Verification items for the finished model (mm, model axes). Face numbers are marked on the shaded views. A direction names the side the tool comes from. Round coordinates to 2 decimals unless told otherwise and drop trailing zeros. Write each loop counter-clockwise with the first axis right and the second up, starting at its lowest first coordinate (ties: lowest second). Pieces come first, ordered by that corner, then holes. Notation, with made-up numbers: (40.5, 44.25) - (60.5, 44.25) arc R22 cw to (60.5, 73.25) - close; hole circle Ø8 at (63.25, -37). An arc over 180 degrees is marked (long way). Answer as a JSON object with one key per item and string values. Group by question number.
1) Section check A-A (y = 4). Enter the section's corners in (x, z) (3 decimals).
2) Section check C-C (y = -8.5). Enter the section's corners in (x, z) (3 decimals), then the cut area to 4 significant figures.
3) Section check D-D (z = -8.5). Enter the section's corners in (x, y), then the cut area to 3 significant figures.
4) Go/stop test with flat-tipped pins: pin 1 Ø4 at (x, z) = (3.5, 12) entering from -Y; pin 2 Ø10 at (x, z) = (8, 4.5) entering from +Y; pin 3 Ø3 at (x, y) = (-26, 3.5) entering from -Z. Record where each tip stops, or that it passes through.
5) Thickness scan on line 1 (X direction, y = 0, z = 21) (3 decimals); line 2 (X direction, y = 5, z = 0) (3 decimals). Record the ranges inside material, lowest first.
6) Mould release check, pull along Z, two halves, no side actions. Record for the marked faces 6, 7 and 8: +Z half, -Z half, draft (parallel to the pull), parting line (faces both ways), or undercut.
7) Section check B-B (z = 10). Enter the section's corners in (x, y).
8) Set-up check for the marked faces 1, 2, 3, 4 and 5: record each of +Z, -Z, +X, -X, +Y, -Y from which the full face is reachable in a straight line by a thin tool's end or side.
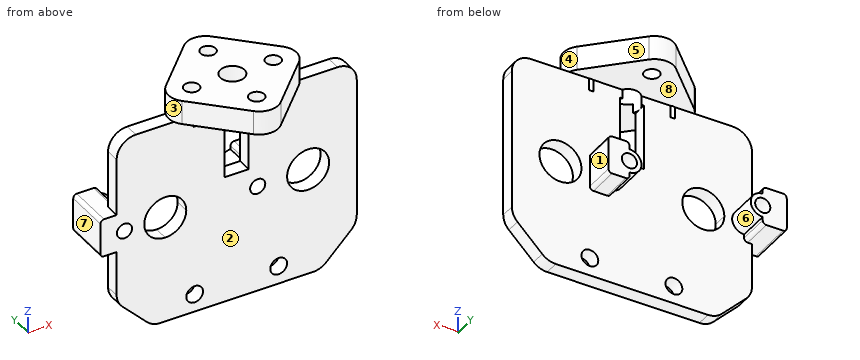
```python
from build123d import *

# Parameters (mm, degrees)
BOSS_EXTRUDE1_DEPTH      = 1.5
BOSS_EXTRUDE1_DEPTH_BACK = 1.5
SKETCH1_W                = 5
SKETCH1_H                = 13.727853371
SKETCH1_R                = 4.375
SKETCH1_R_2              = 1.75
BOSS_EXTRUDE2_DEPTH      = 15
BOSS_EXTRUDE2_DEPTH_BACK = 15
SKETCH2_R                = 1.575
SKETCH2_R_2              = 2.5
CUT_EXTRUDE1_DEPTH       = 7.5
CUT_EXTRUDE2_DEPTH       = 5
BOSS_EXTRUDE3_DEPTH      = 8
BOSS_EXTRUDE3_DEPTH_BACK = 1.5
SKETCH1_4_R              = 1.575
FILLET1_R                = 4
FILLET2_R                = 0.75


with BuildPart() as part:
    # Sketch1 → Boss-Extrude1 (new, two sides: drawn at the far end of the back side and taken through both)
    with BuildSketch(Plane(origin=(0, 0, 0), x_dir=(1, 0, 0), z_dir=(0, 1, 0)).offset(-BOSS_EXTRUDE1_DEPTH_BACK)):
        with BuildLine():
            ThreePointArc((-23.375, 2.5), (-21.607233047, 1.767766953), (-20.875, 0))
            ThreePointArc((-20.875, 0), (-21.607233047, -1.767766953), (-23.375, -2.5))
            Line((-23.375, -2.5), (-23.375, -4))
            Line((-23.375, -4), (-25, -4))
            Line((-25, -4), (-25, -20))
            Line((-25, -20), (25, -20))
            Line((25, -20), (25, 15))
            Line((25, 15), (17.5, 22.5))
            Line((17.5, 22.5), (-17.5, 22.5))
            Line((-17.5, 22.5), (-25, 15))
            Line((-25, 15), (-25, 4))
            Line((-25, 4), (-23.375, 4))
            Line((-23.375, 4), (-23.375, 2.5))
        make_face()
        with Locations((0, -11.238926686)):
            Rectangle(SKETCH1_W, SKETCH1_H, mode=Mode.SUBTRACT)
        with BuildLine():
            ThreePointArc((-10.5, 0), (-14.875, -4.375), (-19.25, 0))
            ThreePointArc((-19.25, 0), (-17.968592168, 3.093592168), (-14.875, 4.375))
            ThreePointArc((-14.875, 4.375), (-11.781407832, 3.093592168), (-10.5, 0))
        make_face(mode=Mode.SUBTRACT)
        with BuildLine():
            ThreePointArc((4.375, -2.5), (2.607233047, -1.767766953), (1.875, 0))
            ThreePointArc((1.875, 0), (2.607233047, 1.767766953), (4.375, 2.5))
            Line((4.375, 2.5), (4.375, 4))
            Line((4.375, 4), (8.75, 4))
            Line((8.75, 4), (8.75, 0))
            Line((8.75, 0), (8.75, -4))
            Line((8.75, -4), (4.375, -4))
            Line((4.375, -4), (4.375, -2.5))
        make_face(mode=Mode.SUBTRACT)
        with Locations(Location((14.875, 0, 0), (0, 0, 270))):
            Circle(SKETCH1_R, mode=Mode.SUBTRACT)
        with Locations(Location((-8.75, 18.75, 0), (0, 0, 270))):
            Circle(SKETCH1_R_2, mode=Mode.SUBTRACT)
        with Locations(Location((8.75, 18.75, 0), (0, 0, 270))):
            Circle(SKETCH1_R_2, mode=Mode.SUBTRACT)
    extrude(amount=BOSS_EXTRUDE1_DEPTH + BOSS_EXTRUDE1_DEPTH_BACK)

    # Sketch1<3> → Boss-Extrude2 (add, two sides: drawn at the far end of the back side and taken through both)
    with BuildSketch(Plane(origin=(0, 0, 0), x_dir=(1, 0, 0), z_dir=(0, 1, 0)).offset(-BOSS_EXTRUDE2_DEPTH_BACK)):
        Polygon((0, -20), (-25, -20), (-25, -25), (25, -25), (25, -20), align=None)
    extrude(amount=BOSS_EXTRUDE2_DEPTH + BOSS_EXTRUDE2_DEPTH_BACK)

    # Sketch2 → Cut-Extrude1 (cut)
    with BuildSketch(Plane.XY.offset(25)):
        with Locations((-8.5, 0)):
            Circle(SKETCH2_R)
        Circle(SKETCH2_R_2)
        with Locations((0, 8.5)):
            Circle(SKETCH2_R)
        with Locations((8.5, 0)):
            Circle(SKETCH2_R)
        with Locations((0, -8.5)):
            Circle(SKETCH2_R)
    extrude(amount=-CUT_EXTRUDE1_DEPTH, mode=Mode.SUBTRACT)

    # Sketch2<3> → Cut-Extrude2 (cut)
    with BuildSketch(Plane.XY.offset(25)):
        Polygon((-25, 0), (-15, 0), (0, 15), (-25, 15), align=None)
        Polygon((25, 15), (0, 15), (15, 0), (0, -15), (25, -15), align=None)
        Polygon((0, -15), (-15, 0), (-25, 0), (-25, -15), align=None)
    extrude(amount=-CUT_EXTRUDE2_DEPTH, mode=Mode.SUBTRACT)

    # Sketch1<4> → Boss-Extrude3 (add, two sides: drawn at the far end of the back side and taken through both)
    # profile 1 of 2: a face of its own
    with BuildSketch(Plane(origin=(0, 0, 0), x_dir=(1, 0, 0), z_dir=(0, 1, 0)).offset(-BOSS_EXTRUDE3_DEPTH_BACK)):
        with BuildLine():
            ThreePointArc((4.375, 2.5), (1.875, 0), (4.375, -2.5))
            Line((4.375, -2.5), (4.375, -4))
            Line((4.375, -4), (8.75, -4))
            Line((8.75, -4), (8.75, 4))
            Line((8.75, 4), (4.375, 4))
            Line((4.375, 4), (4.375, 2.5))
        make_face()
        with Locations(Location((4.375, 0, 0), (0, 0, 270))):
            Circle(SKETCH1_4_R, mode=Mode.SUBTRACT)
    # profile 2 of 2: a face of its own
    with BuildSketch(Plane(origin=(0, 0, 0), x_dir=(1, 0, 0), z_dir=(0, 1, 0)).offset(-BOSS_EXTRUDE3_DEPTH_BACK)):
        with BuildLine():
            ThreePointArc((-23.375, -2.5), (-20.875, 0), (-23.375, 2.5))
            Line((-23.375, 2.5), (-23.375, 4))
            Line((-23.375, 4), (-28.375, 4))
            Line((-28.375, 4), (-28.375, -4))
            Line((-28.375, -4), (-23.375, -4))
            Line((-23.375, -4), (-23.375, -2.5))
        make_face()
        with Locations(Location((-23.375, 0, 0), (0, 0, 270))):
            Circle(SKETCH1_4_R, mode=Mode.SUBTRACT)
    extrude(amount=BOSS_EXTRUDE3_DEPTH + BOSS_EXTRUDE3_DEPTH_BACK)

    # Fillet1
    # the kernel refuses this fillet: 4 mm, written as the material it takes off along each edge
    with BuildSketch(Plane(origin=(15, 0, 35), x_dir=(-0.7071067811865535, -0.7071067811865416, 0), z_dir=(0, 0, -1))) as fillet1_piece_1:
        with BuildLine():
            CenterArc((FILLET1_R, FILLET1_R), FILLET1_R, 180, 90)
            Line((0, FILLET1_R), (0, 0))
            Line((0, 0), (FILLET1_R, 0))
        make_face()
    extrude(amount=15, mode=Mode.SUBTRACT)
    with BuildSketch(Plane(origin=(0, 15, 35), x_dir=(0.7071067811865505, -0.7071067811865446, 0), z_dir=(0, 0, -1))) as fillet1_piece_2:
        with BuildLine():
            CenterArc((FILLET1_R, FILLET1_R), FILLET1_R, 180, 90)
            Line((0, FILLET1_R), (0, 0))
            Line((0, 0), (FILLET1_R, 0))
        make_face()
    extrude(amount=25, mode=Mode.SUBTRACT)
    with BuildSketch(Plane(origin=(25, -11.5, 20), x_dir=(0, 0, -1), z_dir=(0, 1, 0)), Plane(origin=(-25, -11.5, 20), x_dir=(1, 0, 0), z_dir=(0, 1, 0))) as fillet1_piece_3:
        with BuildLine():
            CenterArc((FILLET1_R, FILLET1_R), FILLET1_R, 180, 90)
            Line((0, FILLET1_R), (0, 0))
            Line((0, 0), (FILLET1_R, 0))
        make_face()
    extrude(amount=23, mode=Mode.SUBTRACT)
    with BuildSketch(Plane(origin=(0, -15, 35), x_dir=(0.7071067811865533, 0.7071067811865418, 0), z_dir=(0, 0, -1))) as fillet1_piece_4:
        with BuildLine():
            CenterArc((FILLET1_R, -FILLET1_R), FILLET1_R, 90, 90)
            Line((0, -FILLET1_R), (0, 0))
            Line((0, 0), (FILLET1_R, 0))
        make_face()
    extrude(amount=25, mode=Mode.SUBTRACT)
    with BuildSketch(Plane(origin=(-15, 0, 35), x_dir=(0.7071067811865416, -0.7071067811865536, 0), z_dir=(0, 0, -1))) as fillet1_piece_5:
        with BuildLine():
            CenterArc((FILLET1_R, -FILLET1_R), FILLET1_R, 90, 90)
            Line((0, -FILLET1_R), (0, 0))
            Line((0, 0), (FILLET1_R, 0))
        make_face()
    extrude(amount=15, mode=Mode.SUBTRACT)
    with BuildSketch(Plane(origin=(-25, -5.642135624, -15), x_dir=(0, 0, 1), z_dir=(0, 1, 0)), Plane(origin=(-17.5, -5.642135624, -22.5), x_dir=(-0.7071067811865465, 0, 0.7071067811865487), z_dir=(0, 1, 0)), Plane(origin=(25, 5.642135624, -15), x_dir=(0, 0, 1), z_dir=(0, -1, 0))) as fillet1_piece_6:
        with BuildLine():
            CenterArc((FILLET1_R * 0.414213562373, FILLET1_R), FILLET1_R, 225, 45)
            Line((-FILLET1_R * 0.292893218813, FILLET1_R * 0.292893218813), (0, 0))
            Line((0, 0), (FILLET1_R * 0.414213562373, 0))
        make_face()
    extrude(amount=11.284271247, mode=Mode.SUBTRACT)
    with BuildSketch(Plane(origin=(17.5, -5.642135624, -22.5), x_dir=(0.7071067811865454, 0, 0.7071067811865497), z_dir=(0, 1, 0))) as fillet1_piece_7:
        with BuildLine():
            CenterArc((FILLET1_R * 0.414213562373, -FILLET1_R), FILLET1_R, 90, 45)
            Line((-FILLET1_R * 0.292893218813, -FILLET1_R * 0.292893218813), (0, 0))
            Line((0, 0), (FILLET1_R * 0.414213562373, 0))
        make_face()
    extrude(amount=11.284271247, mode=Mode.SUBTRACT)

    # Fillet2
    fillet2_edges = [part.edges().sort_by_distance(p)[0] for p in [
        (8.75, 4.75, -4),
        (8.75, 4.75, 4),
        (4.375, 4.75, 4),
        (4.375, 4.75, -4),
        (-28.375, 3.25, 4),
        (-28.375, 3.25, -4),
        (-23.375, 4.75, -4),
        (-23.375, 4.75, 4),
    ]]
    fillet(fillet2_edges, radius=FILLET2_R)


solid = part.part
```
Returned:
{
 "1": {"outline": "(-28.375, -3.25) arc R0.75 ccw to (-27.625, -4) - (-24.125, -4) arc R0.75 ccw to (-23.375, -3.25) - (-23.375, -2.5) arc R2.5 ccw to (-23.375, 2.5) - (-23.375, 3.25) arc R0.75 ccw to (-24.125, 4) - (-27.625, 4) arc R0.75 ccw to (-28.375, 3.25) - close; (-11, 20) - (11, 20) - (11, 25) - (-11, 25) - close; (4.375, -3.25) arc R0.75 ccw to (5.125, -4) - (8, -4) arc R0.75 ccw to (8.75, -3.25) - (8.75, 3.25) arc R0.75 ccw to (8, 4) - (5.125, 4) arc R0.75 ccw to (4.375, 3.25) - (4.375, 2.5) arc R2.5 ccw to (4.375, -2.5) - close; hole circle Ø3.15 at (-23.375, 0); hole circle Ø3.15 at (4.375, 0)"},
 "2": {"outline": "(-6.5, 20) - (-1.575, 20) - (-1.575, 25) - (-6.5, 25) - close; (1.575, 20) - (6.5, 20) - (6.5, 25) - (1.575, 25) - close", "area": "49.25 mm2"},
 "3": {"outline": "(-25, -1.5) - (25, -1.5) - (25, 1.5) - (-25, 1.5) - close", "area": "150 mm2"},
 "4": {"pin 1": "y = -1.5", "pin 2": "y = 8", "pin 3": "z = -4"},
 "5": {"line 1": "-13.343 to -10.075, -6.925 to -2.5, 2.5 to 6.925, 10.075 to 13.343", "line 2": "-28.375 to -24.95, -21.8 to -20.875, 1.875 to 2.8, 5.95 to 8.75"},
 "6": {"face 6": "parting line", "face 7": "draft", "face 8": "undercut"},
 "7": {"outline": "(-25, -1.5) - (-2.5, -1.5) - (-2.5, 1.5) - (-25, 1.5) - close; (2.5, -1.5) - (25, -1.5) - (25, 1.5) - (2.5, 1.5) - close"},
 "8": {"face 1": "-Z, +X, +Y", "face 2": "-Z, +X, -X, -Y", "face 3": "+Z, -X", "face 4": "+Z, +X", "face 5": "+Z, +X, +Y"}
}
